Read the model definition and answer for the solid it produces. Units are mm, in the model's axes. A direction names the side the tool comes from. Coordinates: 2 decimals unless noted, no trailing zeros. Loops run counter-clockwise (first coordinate to the right, second up) from the corner with the lowest first, then second, coordinate; pieces in that order, holes last. Notation, with made-up numbers: (-40, -18) - (-3, -18) arc R35 ccw to (-3, 14) - close; hole circle Ø9 at (-32.5, -13). An arc over 180 degrees is marked (long way). Use CSV: the item, a comma, the result in double quotes.
```python
from build123d import *

# Parameters (mm, degrees)
SKETCH5_W           = 25
SKETCH5_H           = 25
BOSS_EXTRUDE3_DEPTH = 15
SKETCH6_R           = 8.5
SKETCH6_W           = 4.441456536
SKETCH6_H           = 0.851518301
SKETCH6_W_2         = 4.412060549
SKETCH6_H_2         = 0.8515183
SKETCH6_W_3         = 4.475416112
SKETCH6_W_4         = 4.837812326
SKETCH6_W_5         = 5.604508377
CUT_EXTRUDE3_DEPTH  = 3


with BuildPart() as part:
    # Sketch5 → Boss-Extrude3 (new body)
    with BuildSketch(Plane.XY):
        with Locations((0.01465692, 0.007301744)):
            Rectangle(SKETCH5_W, SKETCH5_H)
    extrude(amount=BOSS_EXTRUDE3_DEPTH)

    # Sketch6 → Cut-Extrude3 (cut)
    with BuildSketch(Plane.XY.offset(15)):
        Circle(SKETCH6_R)
        with Locations((-10.445228229, 1.72077303)):
            Rectangle(SKETCH6_W, SKETCH6_H)
        with Locations((-10.459926223, 0.199178628)):
            Rectangle(SKETCH6_W_2, SKETCH6_H_2)
        with Locations((-10.451337758, -1.230194922)):
            Rectangle(SKETCH6_W_3, SKETCH6_H_2)
        with Locations((-10.270139651, -2.633825362)):
            Rectangle(SKETCH6_W_4, SKETCH6_H)
        with Locations((-9.909880943, -4.16280996)):
            Rectangle(SKETCH6_W_5, SKETCH6_H)
    extrude(amount=-CUT_EXTRUDE3_DEPTH, mode=Mode.SUBTRACT)


solid = part.part
```
Q1. The part is cut by section A-A on x = 0. Determine the outline of the cut face in (y, z), and give its area (3 significant figures).
Reported:
outline,"(-12.49, 0) - (12.51, 0) - (12.51, 15) - (8.5, 15) - (8.5, 12) - (-8.5, 12) - (-8.5, 15) - (-12.49, 15) - close"
area,"324 mm²"
Q2. Find the intervals of material crossed by probe 1 along Y at (x, z) = (0, 13.1); probe 2 along Z at (x, y) = (0, -5.5); probe 3 along X at (y, z) = (0, 13.55), in increasing order. Write a range as [from, to].
Reported:
probe 1,"y = [-12.49, -8.5], [8.5, 12.51]"
probe 2,"z = [0, 12]"
probe 3,"x = [8.5, 12.51]"
Q3. The part is cut by section B-B on y = 3. Determine the outline of the cut face in (x, z), and give its area (3 significant figures).
Reported:
outline,"(-12.49, 0) - (12.51, 0) - (12.51, 15) - (7.95, 15) - (7.95, 12) - (-7.95, 12) - (-7.95, 15) - (-12.49, 15) - close"
area,"327 mm²"
Q4. For a pull along Y with two mould halves and no side action, classify faces 1 (the face through (-11, 0.625, 14)), 2 (the face through (0, 12.507, 7)), 3 (the face through (0, -12.493, 7)) as +Y half, -Y half, draft (parallel to the pull), parting line (faces both ways), or undercut.
Reported:
face 1,"undercut"
face 2,"+Y half"
face 3,"-Y half"
Q5. A tool of negligible diameter and unlimited length cuts with its end or side. For faces 4 (the face through (-10, -1.656, 14)), 5 (the face through (8.44, 1.01, 13.52)), 6 (the face through (-12.485, 0, 7)), from which of +Z, -Z, +X, -X, +Y, -Y can it reach the whole face along a straight path? Write none if from no direction.
Reported:
face 4,"+Z, -X"
face 5,"+Z"
face 6,"+Z, -Z, -X, +Y, -Y"
